The drawing under review shows one solid part. Ordinate dimensions are in mm from its lowest x, y, z. A direction names the side the tool comes from. Coordinates: 2 decimals unless noted, no trailing zeros. Write each loop counter-clockwise with the first axis right and the second up, starting at its lowest first coordinate (ties: lowest second). Pieces come first, ordered by that corner, then holes.
1) Machinability: for the marked faces 4 and 5, which of the approach directions +Z, -Z, +X, -X, +Y, -Y give a long, thin tool a straight path to every point of the face, cutting with its end or side? Answer none if there is none.
2) Add section D-D, the plane z = 25.5. State the section outline as (x, y) points (1 decimal).
3) Add section B-B, the plane x = 65.5. State the section outline as (y, z) points.
4) For P1, Ø7.5, axis at x = 17.78, y = 12.7, coming from the -Z side; P2, Ø3, axis at x = 71.5, z = 53, coming from the +Y side; P3, Ø10, axis at x = 62.5, y = 24.5, coming from the -Z side, all flat-tipped, find the tip position at first contact; note any pin that passes through.
5) Add section A-A, the plane y = 12.7. State the section outline as (x, z) points (1 decimal).
6) For line 1 (X direction, y = 60, z = 55.5); line 2 (X direction, y = 12, z = 115); line 3 (Y direction, x = 17.78, z = 115.6), list the stretches that pass through material, from the lowest coordinate up.
7) Mouldability with a two-part tool opening along X and no side actions: class the marked faces 1, 2 and 3 as released by +X, released by -X, zero draft, split by the parting line, or undercut.
8) Add section C-C, the plane y = 36. State the section outline as (x, z) points (1 decimal).
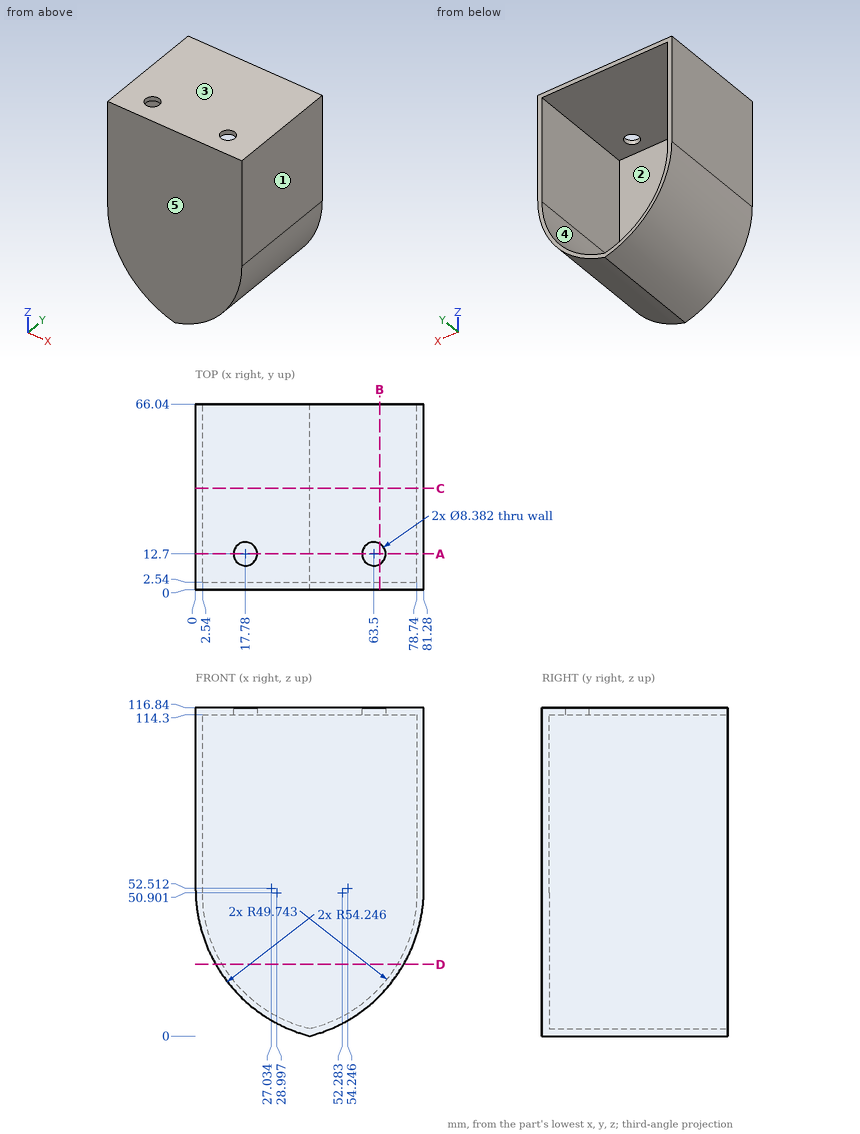
Geometry results:
1. face 4: +Y
1. face 5: +Z, -Z, +X, -X, -Y
2. outline: (7.2, 0) - (74.1, 0) - (74.1, 66) - (71.8, 66) - (71.8, 2.5) - (9.5, 2.5) - (9.5, 66) - (7.2, 66) - close
3. outline: (0, 14.26) - (66.04, 14.26) - (66.04, 17.11) - (2.54, 17.11) - (2.54, 114.3) - (9.02, 114.3) - (9.02, 116.84) - (0, 116.84) - close; (16.38, 114.3) - (66.04, 114.3) - (66.04, 116.84) - (16.38, 116.84) - close
4. P1: stops at z = 9.24
4. P2: stops at y = 2.54
4. P3: stops at z = 7.63
5. outline: (0, 52.5) arc R54.2 ccw to (40.6, 0) arc R54.2 ccw to (81.3, 52.5) - (81.3, 116.8) - (67.7, 116.8) - (67.7, 114.3) - (78.7, 114.3) - (78.7, 50.9) arc R49.7 cw to (40.6, 2.5) arc R49.7 cw to (2.5, 50.9) - (2.5, 114.3) - (13.6, 114.3) - (13.6, 116.8) - (0, 116.8) - close; (22, 114.3) - (59.3, 114.3) - (59.3, 116.8) - (22, 116.8) - close
6. line 1: x = 0 to 2.54, 78.74 to 81.28
6. line 2: x = 0 to 13.65, 21.91 to 59.37, 67.63 to 81.28
6. line 3: y = 0 to 8.51, 16.89 to 66.04
7. face 1: released by +X
7. face 2: undercut
7. face 3: zero draft
8. outline: (0, 52.5) arc R54.2 ccw to (40.6, 0) arc R54.2 ccw to (81.3, 52.5) - (81.3, 116.8) - (0, 116.8) - close; hole (2.5, 50.9) arc R49.7 ccw to (40.6, 2.5) arc R49.7 ccw to (78.7, 50.9) - (78.7, 114.3) - (2.5, 114.3) - close
